Source: CAD feature listing. Evaluate the final solid. Frame: model axes, mm. Face numbers are marked on the shaded views. A direction names the side the tool comes from. Give positions to 0.01 mm unless a question says otherwise; leave off trailing zeros. Loops run counter-clockwise (first coordinate to the right, second up) from the corner with the lowest first, then second, coordinate; pieces in that order, holes last. Notation, with made-up numbers: (71, 86.5) - (125, 86.5) arc R25 cw to (125, 108.5) - close; hole circle Ø9 at (7, 84.5). An arc over 180 degrees is marked (long way). Write each question's results on one line, items separated by ' | '. Start each with the question number.
(1) Cut plane B-B on z = 0. Return the cut outline in (x, y), then the cut area to 3 significant figures.
(2) Reachability of the marked faces 1, 2 and 3 from +Z, -Z, +X, -X, +Y, -Y: full face, straight path, thin tool, end or side. Return the list, or none.
(3) Contact query for flat-ended pins moving along their axis: pin 1 (12 mm diameter, centred on x = 8.5, y = 16, fed in from -Z); pin 2 (3 mm diameter, centred on y = 157, z = -19.5, fed in from -X); pin 3 (5 mm diameter, centred on x = -7.5, z = -6.5, fed in from +Y). Output: stop coordinate, or through.
(4) Cut plane C-C on z = -30.5. Return the cut outline in (x, y).
(5) Material intervals for line 1 along Y through (x, z) = (2, 0); line 2 along X through (y, z) = (136, -19); line 3 along Z through (x, y) = (-4.5, 141), sorted ascending. Write a range as [from, to].
(6) Pull-direction query (Z, two-part tool) for the marked faces 4, 5 and 6; classes: pulls with the +Z half, pulls with the -Z half, needs draft (parallel to the pull), parting line crosses it, or undercut.
(7) Cut plane A-A on y = 45. Return the cut outline in (x, z), then the cut area to 3 significant figures.
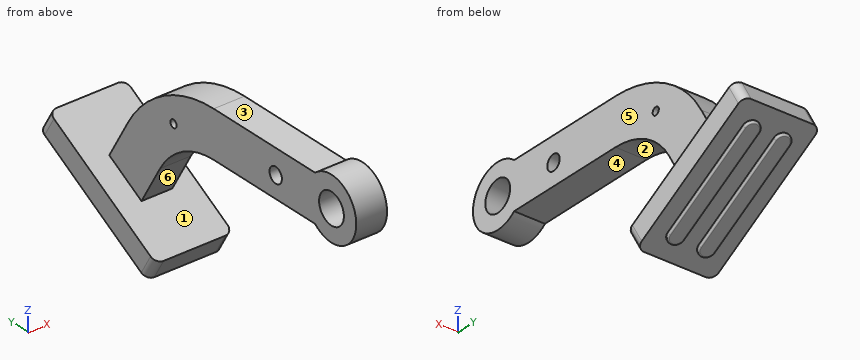
from build123d import *

# Parameters (mm, degrees)
SKETCH3_R           = 10
SKETCH3_R_2         = 5
SKETCH3_R_3         = 2.5
BOSS_EXTRUDE1_DEPTH = 10
BOSS_EXTRUDE2_DEPTH = 25
FILLET1_R           = 5
BOSS_EXTRUDE4_DEPTH = 2
FILLET6_R           = 1


with BuildPart() as part:
    # Sketch3 → Boss-Extrude1 (new body, symmetric)
    with BuildSketch(Plane(origin=(0, 0, 0), x_dir=(0, 0, -1), z_dir=(1, 0, 0))):
        with BuildLine():
            Line((65.980762114, 153.301270189), (50.980762114, 179.282032303))
            Line((50.980762114, 179.282032303), (25, 164.282032303))
            ThreePointArc((25, 164.282032303), (-4.282032303, 135), (-15, 95))
            Line((-15, 95), (-15, 13.228756555))
            ThreePointArc((-15, 13.228756555), (0, -20), (15, 13.228756555))
            Line((15, 13.228756555), (15, 95))
            ThreePointArc((15, 95), (21.698729811, 120), (40, 138.301270189))
            Line((40, 138.301270189), (65.980762114, 153.301270189))
        make_face()
        Circle(SKETCH3_R, mode=Mode.SUBTRACT)
        with Locations((1.032464383, 45)):
            Circle(SKETCH3_R_2, mode=Mode.SUBTRACT)
        with Locations((8.708348754, 127.5)):
            Circle(SKETCH3_R_3, mode=Mode.SUBTRACT)
    extrude(amount=BOSS_EXTRUDE1_DEPTH, both=True)

    # Sketch3_3 → Boss-Extrude2 (add, symmetric)
    with BuildSketch(Plane(origin=(0, 0, 0), x_dir=(0, 0, -1), z_dir=(1, 0, 0))):
        Polygon((33.480762114, 209.592921435), (46.47114317, 217.092921435), (96.47114317, 130.490381057), (83.480762114, 122.990381057), align=None)
    extrude(amount=BOSS_EXTRUDE2_DEPTH, both=True)

    # Fillet1
    fillet1_edges = [part.edges().sort_by_distance(p)[0] for p in [
        (25, 213.342921435, -39.975952642),
        (25, 126.740381057, -89.975952642),
        (-25, 213.342921435, -39.975952642),
        (-25, 126.740381057, -89.975952642),
    ]]
    fillet(fillet1_edges, radius=FILLET1_R)

    # Sketch6 → Boss-Extrude4 (add)
    with BuildSketch(Plane(origin=(0, 74.395825623, -128.85734985), x_dir=(-1, 0, 0), z_dir=(0, 0.5, -0.866025404))):
        with BuildLine():
            Line((-5, 149.77241336), (-5, 79.77241336))
            ThreePointArc((-5, 79.77241336), (-10, 74.77241336), (-15, 79.77241336))
            Line((-15, 79.77241336), (-15, 149.77241336))
            ThreePointArc((-15, 149.77241336), (-10, 154.77241336), (-5, 149.77241336))
        make_face()
        with BuildLine():
            Line((15, 149.77241336), (15, 79.77241336))
            ThreePointArc((15, 79.77241336), (10, 74.77241336), (5, 79.77241336))
            Line((5, 79.77241336), (5, 149.77241336))
            ThreePointArc((5, 149.77241336), (10, 154.77241336), (15, 149.77241336))
        make_face()
    extrude(amount=BOSS_EXTRUDE4_DEPTH)

    # Fillet6
    fillet6_edges = [part.edges().sort_by_distance(p)[0] for p in [
        (10, 209.432667397, -53.203193978),
        (15, 174.791651246, -73.203193978),
        (10, 140.150635095, -93.203193978),
        (5, 174.791651246, -73.203193978),
        (-10, 209.432667397, -53.203193978),
        (-5, 174.791651246, -73.203193978),
        (-10, 140.150635095, -93.203193978),
        (-15, 174.791651246, -73.203193978),
    ]]
    fillet(fillet6_edges, radius=FILLET6_R)


solid = part.part
Ans:
1) outline: (-10, -20) - (10, -20) - (10, -10) - (-10, -10) - close; (-10, 10) - (10, 10) - (10, 40.11) - (-10, 40.11) - close; (-10, 49.89) - (10, 49.89) - (10, 141.64) - (-10, 141.64) - close | area: 2,640 mm^2
2) face 1: none | face 2: +X, -X | face 3: +Z, +X, -X, +Y
3) pin 1: z = -17.32 | pin 2: x = -10 | pin 3: y = 152.13
4) outline: (-10, 131.19) - (10, 131.19) - (10, 167.46) - (-10, 167.46) - close
5) line 1: [-20, -10], [10, 40.11], [49.89, 141.64] | line 2: [-10, 10] | line 3: [-90.4, -73.08], [-44.67, 0.45]
6) face 4: pulls with the -Z half | face 5: needs draft | face 6: undercut
7) outline: (-10, -15) - (10, -15) - (10, -6.03) - (-10, -6.03) - close; (-10, 3.97) - (10, 3.97) - (10, 15) - (-10, 15) - close | area: 400 mm^2
